Autodesk Inventor part; units mm, degrees
ref_plane "YZ Plane" through (0, 0, 0) normal (1, 0, 0) x (0, 1, 0)
ref_plane "XZ Plane" through (0, 0, 0) normal (0, 1, 0) x (-1, 0, 0)
ref_plane "XY Plane" through (0, 0, 0) normal (0, 0, 1) x (1, 0, 0)
sketch "Skizze1" plane through (0, 0, 0) normal (0, 0, 1) x (1, 0, 0)
  circle A0 centre (0, 0) radius 7.5
  circle A1 centre (0, 0) radius 10
  line L0 (0, 0) -> (-10, 0)
  line L1 (0, 0) -> (0, -10)
  point P0 (0, -7.5)
  point P1 (-7.5, 0)
  dimension "d0" = 15
  dimension "d1" = 20
extrude "Extrusion1" add sketch "Skizze1" along normal blind 4 contours A0 L0 A1 L1 picked at (-8.9972, 1.396)
sketch "Skizze2" plane through (-10, 0, 0) normal (0, -1, 0) x (1, 0, 0)
  line L0 (2.5, 0) -> (2.5, 4) construction
  line L1 (2.5, 2) -> (4, 2) construction
  line L2 (4, 2) -> (2.5, 4)
  line L3 (20, 4) -> (0, 4)
  line L4 (4, 2) -> (2.5, 0)
  line L5 (2.5, 0) -> (2.5, 4)
  line L6 (10, -0.8) -> (10, 4.8)
  point P0 (10, 0)
  point P1 (10, 4)
  dimension "d4" = 1.5
revolve "Umdrehung1" add sketch "Skizze2" angle 270 about axis through (0, 0, -10) along (0, 0, -1)
properties part number "C-ClipV1"
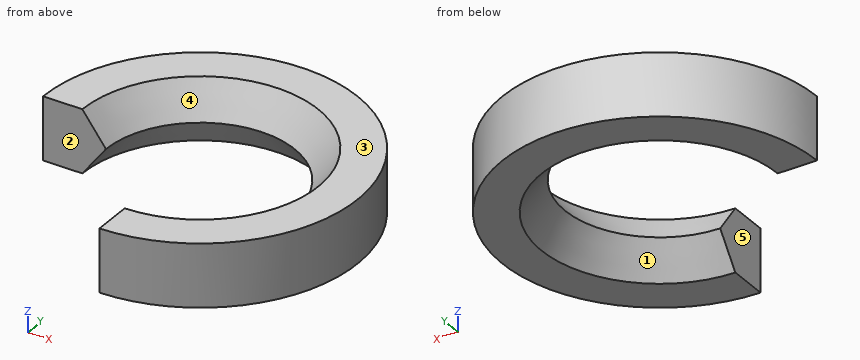
Can you work these out from the model? Positions are in its coordinate system, mm. Face numbers are marked on the shaded views. A direction names the side the tool comes from. Round coordinates to 2 decimals unless told otherwise and drop trailing zeros. Loops run counter-clockwise (first coordinate to the right, second up) from the corner with the lowest first, then second, coordinate; pieces in that order, holes last. Notation, with made-up numbers: M 25,36.5 L 37,36.5 A23 cw 37,61.5 Z; hole C 87,46.5 d2. An arc over 180 degrees is marked long. Answer as a JSON object with one key per item and string values. Group by question number.
Q1. Please list where these lines run through material, in increasing order: L1, parallel to Y at x = 2.5, z = 2.3; L2, parallel to Y at x = 3.75, z = 2.2; L3, parallel to X at y = 4.5, z = 2.05.
Q2. Imagine slicing it at B-B, the plane z = 3.4. Please give me the cut outline in (x, y), then the cut area to 3 significant figures.
Q3. Will these pins go through, and if not, where does the flat tip stop? pin 1 (12 mm diameter, centred on x = -7.5, y = 7, fed in from -Z); pin 2 (1 mm diameter, centred on x = -6, z = 1, fed in from +Y); pin 3 (4 mm diameter, centred on x = 4.5, y = 1, fed in from +Z); pin 4 (1.2 mm diameter, centred on x = -8.5, z = 1.5, fed in from -Y).
Q4. Imagine slicing it at A-A, the plane z = 0.8. Please give me the cut outline in (x, y), then the cut area to 3 significant figures.
Q5. We'd pull the mould along Y, two halves only. Please class the marked faces 1, 2 and 3: +Y half, -Y half, draft (parallel to the pull), parting line (faces both ways), or undercut.
Q6. On a 3-axis mill with a long thin cutter (end or side, diameter ignored), from which of +Z, -Z, +X, -X, +Y, -Y can I reach the whole of each face in a straight line? I mean the marked faces 4 and 5. Say none if no direction works.
Findings:
{
 "1": {"L1": "y = -9.68 to -5.7, 5.7 to 9.68", "L2": "y = -9.27 to -4.87, 4.87 to 9.27", "L3": "x = -8.93 to -4.03, 4.03 to 8.93"},
 "2": {"outline": "M -10,0 L -7.05,0 A7.05 cw long 0,-7.05 L 0,-10 A10 ccw long Z", "area": "119 mm2"},
 "3": {"pin 1": "stops at z = 0", "pin 2": "stops at y = 8.35", "pin 3": "stops at z = 2.81", "pin 4": "stops at y = 0"},
 "4": {"outline": "M -10,0 L -6.9,0 A6.9 cw long 0,-6.9 L 0,-10 A10 ccw long Z", "area": "123 mm2"},
 "5": {"face 1": "undercut", "face 2": "-Y half", "face 3": "draft"},
 "6": {"face 4": "+Z", "face 5": "+Z, -Z, -X, -Y"}
}
